The model under review builds one solid part; all positions refer to its coordinate system, in mm. Face numbers are marked on the shaded views. A direction names the side the tool comes from. Give positions to 0.01 mm unless a question says otherwise; leave off trailing zeros. Loops run counter-clockwise (first coordinate to the right, second up) from the corner with the lowest first, then second, coordinate; pieces in that order, holes last. Notation, with made-up numbers: M -26.5,-38 L 10.5,-38 A21 cw 10.5,-24 Z; hole C -25.75,51 d7. An arc over 180 degrees is marked long. Put each result on its own line as item: value. Start each with the question number.
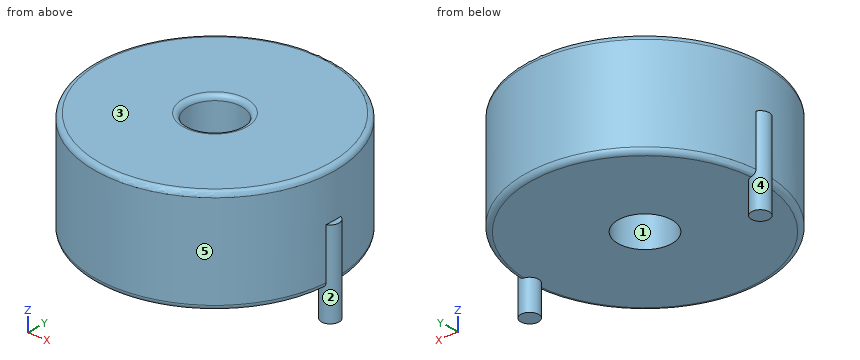
```python
from build123d import *

# Parameters (mm, degrees)
SKETCH001_R       = 0.9
PAD001_DEPTH      = 5.25
PAD001_DEPTH_BACK = 3.5
SKETCH_R          = 12.2
SKETCH_R_2        = 2.75
PAD_DEPTH         = 10.5
FILLET_R          = 0.5


with BuildPart() as pad001:
    # Sketch001 → Pad001 (new body, two sides)
    with BuildSketch(Plane.XY.offset(0.5)) as pad001_sk:
        Circle(SKETCH001_R)
        with Locations((23.7, 0)):
            Circle(SKETCH001_R)
    extrude(amount=PAD001_DEPTH)
    extrude(pad001_sk.sketch, amount=-PAD001_DEPTH_BACK)


with BuildPart() as obj1:
    # Sketch → Pad (new body)
    with BuildSketch(Plane.XY.offset(0.1)):
        with Locations((11.85, 0)):
            Circle(SKETCH_R)
        with Locations((11.85, 0)):
            Circle(SKETCH_R_2, mode=Mode.SUBTRACT)
    extrude(amount=PAD_DEPTH)

    # Fillet
    fillet_edges = [obj1.edges().sort_by_distance(p)[0] for p in [
        (9.1, 0, 10.6),
        (-0.35, 0, 10.6),
        (-0.35, 0, 0.1),
    ]]
    fillet(fillet_edges, radius=FILLET_R)

    # obj1: union Pad001
    add(pad001.part)


solid = obj1.part
```
Item 1: Consider section A-A, the plane y = 0. Write out the cut boundary in (x, z).
Item 2: To check wall thickness, follow L1, parallel to Y at x = 11.85, z = 8.25; L2, parallel to Z at x = 6, y = 3.75; L3, parallel to Y at x = 2.5, z = 6. State the ranges of each line that lie inside material, in increasing order. Write a range as [from, to].
Item 3: Tool access review of the marked faces 1 and 2: name each direction out of +Z, -Z, +X, -X, +Y, -Y from which nothing blocks a thin tool from reaching the whole face with its end or side.
Item 4: Clearance check with flat-ended pins moving along their axes: pin 1 Ø6 at (y, z) = (9, 7.5) entering from +X; pin 2 Ø3 at (x, y) = (18.5, -2) entering from -Z; pin 3 Ø4 at (x, z) = (16.5, 7) entering from -Y; pin 4 Ø3.5 at (x, y) = (11.85, 0) entering from +Z. State where each tip first meets the part, or that it passes through.
Item 5: Consider section B-B, the plane x = 11.85. Write out the cut boundary in (y, z).
Item 6: Consider section C-C, the plane z = 5. Write out the cut boundary in (x, y).
Item 7: Consider section D-D, the plane z = -1.25. Write out the cut boundary in (x, y), plus the area to 3 significant figures.
Item 8: Draft analysis for pull direction X (two halves, no side actions). For the marked faces 3, 4 and 5, state which applies: +X half, -X half, draft (parallel to the pull), parting line (faces both ways), or undercut.
Report:
1. outline: M -0.9,-3 L 0.9,-3 L 0.9,0.1 L 9.1,0.1 L 9.1,10.1 A0.5 ccw 8.6,10.6 L 0.15,10.6 A0.5 ccw -0.35,10.1 L -0.35,5.75 L -0.9,5.75 Z; M 14.6,0.1 L 22.8,0.1 L 22.8,-3 L 24.6,-3 L 24.6,5.75 L 24.05,5.75 L 24.05,10.1 A0.5 ccw 23.55,10.6 L 15.1,10.6 A0.5 ccw 14.6,10.1 Z
2. L1: [-12.2, -2.75], [2.75, 12.2]
2. L2: [0.1, 10.6]
2. L3: [-7.84, 7.84]
3. face 1: +Z, -Z
3. face 2: -Z
4. pin 1: x = 22.47
4. pin 2: z = 0.1
4. pin 3: y = -11.91
4. pin 4: through
5. outline: M -12.2,0.6 A0.5 ccw -11.7,0.1 L -2.75,0.1 L -2.75,10.1 A0.5 ccw -3.25,10.6 L -11.7,10.6 A0.5 ccw -12.2,10.1 Z; M 2.75,0.1 L 11.7,0.1 A0.5 ccw 12.2,0.6 L 12.2,10.1 A0.5 ccw 11.7,10.6 L 3.25,10.6 A0.5 ccw 2.75,10.1 Z
6. outline: M -0.32,-0.84 A12.2 ccw 24.02,-0.84 A0.9 ccw 24.02,0.84 A12.2 ccw -0.32,0.84 A0.9 ccw Z; hole C 11.85,0 d5.5
7. outline: C 0,0 d1.8; C 23.7,0 d1.8
7. area: 5.09 mm²
8. face 3: draft
8. face 4: undercut
8. face 5: parting line
